For this review, take the finished solid that the model builds, in its own axes (mm). A direction names the side the tool comes from. Coordinates: 2 decimals unless noted, no trailing zeros. Loops run counter-clockwise (first coordinate to the right, second up) from the corner with the lowest first, then second, coordinate; pieces in that order, holes last. Notation, with made-up numbers: (16.5, 46) - (67.5, 46) arc R10 cw to (67.5, 59) - close; hole circle Ø8 at (25, 68.5). An arc over 180 degrees is marked (long way). Answer as a JSON object with one key per item and string values. Group by question number.
Item 1: Tool access review of faces 4 (the flat face through (3, -29, 12)), 5 (the flat face through (8, -26.3, 10.7)), 6 (the cylindrical face through (-14.985, 0.66, 12.395)): name each direction out of +Z, -Z, +X, -X, +Y, -Y from which nothing blocks a thin tool from reaching the whole face with its end or side.
Item 2: We need section D-D (y = -12.5). Give the boundary of the cut face in (x, z).
Item 3: We need section A-A (y = 0). Give the boundary of the cut face in (x, z), then the cut area to 3 significant figures.
Item 4: Mouldability with a two-part tool opening along X and no side actions: class faces 1 (the flat face through (3, 29, 12)), 2 (the cylindrical face through (14.068, -14.216, 12.395)), 3 (the flat face through (18, 21, 5)) as released by +X, released by -X, zero draft, split by the parting line, or undercut.
Item 5: We need section C-C (z = 12.5). State how many separate pieces and enclosed holes the cut face has, then the cut area to 3 significant figures.
Item 6: Clearance check with flat-ended pins moving along their axes: pin 1 (7.5 mm diameter, centred on y = -31, z = 9.5, fed in from -X); pin 2 (5 mm diameter, centred on y = 26.6, z = 12.5, fed in from +X); pin 3 (3 mm diameter, centred on y = -17, z = 10, fed in from -X); pin 4 (6 mm diameter, centred on x = -12, y = -19, fed in from +Z). State where each tip first meets the part, or that it passes through.
Item 7: To check wall thickness, follow line 1 (Y direction, x = -23, z = 10); line 2 (X direction, y = 6.65, z = 12.5). State the ranges of each line that lie inside material, in increasing order.
from build123d import *

# Parameters (mm, degrees)
SKETCH2_R           = 35
SKETCH2_R_2         = 5
BOSS_EXTRUDE1_DEPTH = 5
SKETCH3_R           = 20
SKETCH3_R_2         = 15
BOSS_EXTRUDE3_DEPTH = 15
SKETCH4_R           = 1.6
CUT_EXTRUDE1_DEPTH  = 59.940648113
CIRPATTERN1_COUNT   = 4
SKETCH5_R           = 1.9
SKETCH5_R_2         = 1.25
CUT_EXTRUDE2_DEPTH  = 52.720402164


with BuildPart() as part:
    # Sketch2 → Boss-Extrude1 (new body)
    with BuildSketch(Plane.XY):
        Circle(SKETCH2_R)
        Circle(SKETCH2_R_2, mode=Mode.SUBTRACT)
    extrude(amount=BOSS_EXTRUDE1_DEPTH)

    # Sketch3 → Boss-Extrude3 (add)
    # profile 1 of 9: a face of its own
    with BuildSketch(Plane.XY.offset(5)):
        with BuildLine():
            ThreePointArc((-3, -19.773719933), (-5.547149112, -19.215335978), (-8, -18.33030278))
            Line((-8, -18.33030278), (-8, -34.073450075))
            ThreePointArc((-8, -34.073450075), (-5.514444475, -34.562854369), (-3, -34.871191548))
            Line((-3, -34.871191548), (-3, -19.773719933))
        make_face()
    # profile 2 of 9: a face of its own
    with BuildSketch(Plane.XY.offset(5)):
        with BuildLine():
            Line((8, -34.073450075), (8, -18.33030278))
            ThreePointArc((8, -18.33030278), (5.547149112, -19.215335978), (3, -19.773719933))
            Line((3, -19.773719933), (3, -34.871191548))
            ThreePointArc((3, -34.871191548), (5.514444475, -34.562854369), (8, -34.073450075))
        make_face()
    # profile 3 of 9: a face of its own
    with BuildSketch(Plane.XY.offset(5)):
        with BuildLine():
            Line((34.871191548, -3), (19.773719933, -3))
            ThreePointArc((19.773719933, -3), (19.215335978, -5.547149112), (18.33030278, -8))
            Line((18.33030278, -8), (34.073450075, -8))
            ThreePointArc((34.073450075, -8), (34.562854369, -5.514444475), (34.871191548, -3))
        make_face()
    # profile 4 of 9: a face of its own
    with BuildSketch(Plane.XY.offset(5)):
        with BuildLine():
            Line((34.073450075, 8), (18.33030278, 8))
            ThreePointArc((18.33030278, 8), (19.215335978, 5.547149112), (19.773719933, 3))
            Line((19.773719933, 3), (34.871191548, 3))
            ThreePointArc((34.871191548, 3), (34.562854369, 5.514444475), (34.073450075, 8))
        make_face()
    # profile 5 of 9: a face of its own
    with BuildSketch(Plane.XY.offset(5)):
        with BuildLine():
            Line((3, 34.871191548), (3, 19.773719933))
            ThreePointArc((3, 19.773719933), (5.547149112, 19.215335978), (8, 18.33030278))
            Line((8, 18.33030278), (8, 34.073450075))
            ThreePointArc((8, 34.073450075), (5.514444475, 34.562854369), (3, 34.871191548))
        make_face()
    # profile 6 of 9: a face of its own
    with BuildSketch(Plane.XY.offset(5)):
        with BuildLine():
            ThreePointArc((-8, 18.33030278), (-5.547149112, 19.215335978), (-3, 19.773719933))
            Line((-3, 19.773719933), (-3, 34.871191548))
            ThreePointArc((-3, 34.871191548), (-5.514444475, 34.562854369), (-8, 34.073450075))
            Line((-8, 34.073450075), (-8, 18.33030278))
        make_face()
    # profile 7 of 9: a face of its own
    with BuildSketch(Plane.XY.offset(5)):
        with BuildLine():
            ThreePointArc((-19.773719933, 3), (-19.215335978, 5.547149112), (-18.33030278, 8))
            Line((-18.33030278, 8), (-34.073450075, 8))
            ThreePointArc((-34.073450075, 8), (-34.562854369, 5.514444475), (-34.871191548, 3))
            Line((-34.871191548, 3), (-19.773719933, 3))
        make_face()
    # profile 8 of 9: a face of its own
    with BuildSketch(Plane.XY.offset(5)):
        with BuildLine():
            ThreePointArc((-18.33030278, -8), (-19.215335978, -5.547149112), (-19.773719933, -3))
            Line((-19.773719933, -3), (-34.871191548, -3))
            ThreePointArc((-34.871191548, -3), (-34.562854369, -5.514444475), (-34.073450075, -8))
            Line((-34.073450075, -8), (-18.33030278, -8))
        make_face()
    # profile 9 of 9: a face of its own
    with BuildSketch(Plane.XY.offset(5)):
        Circle(SKETCH3_R)
        Circle(SKETCH3_R_2, mode=Mode.SUBTRACT)
    extrude(amount=BOSS_EXTRUDE3_DEPTH)

    # Sketch4 → Cut-Extrude1 (cut, through all)
    with BuildSketch(Plane.ZY.offset(8)):
        with Locations((12.5, 26.596250524)):
            Circle(SKETCH4_R)
    cut_extrude1 = extrude(amount=-CUT_EXTRUDE1_DEPTH, mode=Mode.SUBTRACT)

    # CirPattern1: Cut-Extrude1 ×4 about axis
    cirpattern1_axis = Axis((0, 0, 20), (0, 0, -1))
    for i in range(1, CIRPATTERN1_COUNT):
        add(cut_extrude1.rotate(cirpattern1_axis, i * 360 / CIRPATTERN1_COUNT), mode=Mode.SUBTRACT)

    # Sketch5 → Cut-Extrude2 (cut, through all)
    with BuildSketch(Plane.XY.offset(5)):
        with Locations((19.405170255, 19.413249431)):
            Circle(SKETCH5_R)
        with Locations((-19.525765468, -19.291950885)):
            Circle(SKETCH5_R_2)
    extrude(amount=-CUT_EXTRUDE2_DEPTH, mode=Mode.SUBTRACT)


solid = part.part
Check sheet entries:
{
 "1": {"face 4": "+Z, -Y", "face 5": "+Z, +X, -Y", "face 6": "+Z"},
 "2": {"outline": "(-32.69, 0) - (32.69, 0) - (32.69, 5) - (15.61, 5) - (15.61, 20) - (8.29, 20) - (8.29, 5) - (-8.29, 5) - (-8.29, 20) - (-15.61, 20) - (-15.61, 5) - (-32.69, 5) - close"},
 "3": {"outline": "(-35, 0) - (-5, 0) - (-5, 5) - (-15, 5) - (-15, 20) - (-20, 20) - (-20, 5) - (-35, 5) - close; (5, 0) - (35, 0) - (35, 5) - (20, 5) - (20, 20) - (15, 20) - (15, 5) - (5, 5) - close", "area": "450 mm2"},
 "4": {"face 1": "undercut", "face 2": "released by +X", "face 3": "zero draft"},
 "5": {"separate pieces": "9", "enclosed holes": "1", "area": "1,040 mm2"},
 "6": {"pin 1": "stops at x = -8", "pin 2": "stops at x = 8", "pin 3": "stops at x = -12.64", "pin 4": "stops at z = 20"},
 "7": {"line 1": "y = -8 to -3, 3 to 8", "line 2": "x = -34.36 to -28.2, -25 to -13.45, 13.45 to 25, 28.2 to 34.36"}
}
